```python
from build123d import *

# Parameters (mm, degrees)
F0_R      = 38.1036206278
F1_DEPTH  = 25
F2_COUNT  = 24
F3_DEPTH  = 35
F4_R      = 5
F5_SIZE   = 5
F7_DEPTH  = 50
F8_T      = -2.5
F10_DEPTH = 25
F11_R     = 7.6453811345
F12_DEPTH = 50


with BuildPart() as f1:
    # F0 (on Front) → F1 (new body)
    with BuildSketch(Plane.XZ):
        with BuildLine():
            ThreePointArc((-7.8842675869, 53.139290225), (-35.0884247435, -40.6785974441), (53.721, 0))
            ThreePointArc((53.721, 0), (38.2966086664, 37.6738052983), (0.8807473744, 53.7137796572))
            ThreePointArc((0.8807473744, 53.7137796572), (-3.5135215054, 53.6059792153), (-7.8842675869, 53.139290225))
        make_face()
        Circle(F0_R, mode=Mode.SUBTRACT)
        with BuildLine():
            ThreePointArc((-7.8842675869, 53.139290225), (-3.5135215054, 53.6059792153), (0.8807473744, 53.7137796572))
            ThreePointArc((0.8807473744, 53.7137796572), (0.6904629861, 56.2382962215), (0, 58.674))
            ThreePointArc((0, 58.674), (-1.2045880723, 61.1890122015), (-2.8564405638, 63.4357213824))
            ThreePointArc((-2.8564405638, 63.4357213824), (-4.0797358778, 62.2447411623), (-5.448019844, 63.2658603022))
            ThreePointArc((-5.448019844, 63.2658603022), (-6.792486114, 60.822762014), (-7.6584938023, 58.1720357962))
            ThreePointArc((-7.6584938023, 58.1720357962), (-8.0251266423, 55.6670462968), (-7.8842675869, 53.139290225))
        make_face()
    extrude(amount=F1_DEPTH)


with BuildPart() as f2_1:
    # F2: instance of F1
    add(f1.part.rotate(Axis((0, 0, 0), (0, 1, 0)), 1 * 360 / F2_COUNT))


with BuildPart() as f2_2:
    # F2: instance of F1
    add(f1.part.rotate(Axis((0, 0, 0), (0, 1, 0)), 2 * 360 / F2_COUNT))


with BuildPart() as f2_3:
    # F2: instance of F1
    add(f1.part.rotate(Axis((0, 0, 0), (0, 1, 0)), 3 * 360 / F2_COUNT))


with BuildPart() as f2_4:
    # F2: instance of F1
    add(f1.part.rotate(Axis((0, 0, 0), (0, 1, 0)), 4 * 360 / F2_COUNT))


with BuildPart() as f2_5:
    # F2: instance of F1
    add(f1.part.rotate(Axis((0, 0, 0), (0, 1, 0)), 5 * 360 / F2_COUNT))


with BuildPart() as f2_6:
    # F2: instance of F1
    add(f1.part.rotate(Axis((0, 0, 0), (0, 1, 0)), 6 * 360 / F2_COUNT))


with BuildPart() as f2_7:
    # F2: instance of F1
    add(f1.part.rotate(Axis((0, 0, 0), (0, 1, 0)), 7 * 360 / F2_COUNT))


with BuildPart() as f2_8:
    # F2: instance of F1
    add(f1.part.rotate(Axis((0, 0, 0), (0, 1, 0)), 8 * 360 / F2_COUNT))


with BuildPart() as f2_9:
    # F2: instance of F1
    add(f1.part.rotate(Axis((0, 0, 0), (0, 1, 0)), 9 * 360 / F2_COUNT))


with BuildPart() as f2_10:
    # F2: instance of F1
    add(f1.part.rotate(Axis((0, 0, 0), (0, 1, 0)), 10 * 360 / F2_COUNT))


with BuildPart() as f2_11:
    # F2: instance of F1
    add(f1.part.rotate(Axis((0, 0, 0), (0, 1, 0)), 11 * 360 / F2_COUNT))


with BuildPart() as f2_12:
    # F2: instance of F1
    add(f1.part.rotate(Axis((0, 0, 0), (0, 1, 0)), 12 * 360 / F2_COUNT))


with BuildPart() as f2_13:
    # F2: instance of F1
    add(f1.part.rotate(Axis((0, 0, 0), (0, 1, 0)), 13 * 360 / F2_COUNT))


with BuildPart() as f2_14:
    # F2: instance of F1
    add(f1.part.rotate(Axis((0, 0, 0), (0, 1, 0)), 14 * 360 / F2_COUNT))


with BuildPart() as f2_15:
    # F2: instance of F1
    add(f1.part.rotate(Axis((0, 0, 0), (0, 1, 0)), 15 * 360 / F2_COUNT))


with BuildPart() as f2_16:
    # F2: instance of F1
    add(f1.part.rotate(Axis((0, 0, 0), (0, 1, 0)), 16 * 360 / F2_COUNT))


with BuildPart() as f2_17:
    # F2: instance of F1
    add(f1.part.rotate(Axis((0, 0, 0), (0, 1, 0)), 17 * 360 / F2_COUNT))


with BuildPart() as f2_18:
    # F2: instance of F1
    add(f1.part.rotate(Axis((0, 0, 0), (0, 1, 0)), 18 * 360 / F2_COUNT))


with BuildPart() as f2_19:
    # F2: instance of F1
    add(f1.part.rotate(Axis((0, 0, 0), (0, 1, 0)), 19 * 360 / F2_COUNT))


with BuildPart() as f2_20:
    # F2: instance of F1
    add(f1.part.rotate(Axis((0, 0, 0), (0, 1, 0)), 20 * 360 / F2_COUNT))


with BuildPart() as f2_21:
    # F2: instance of F1
    add(f1.part.rotate(Axis((0, 0, 0), (0, 1, 0)), 21 * 360 / F2_COUNT))


with BuildPart() as f2_22:
    # F2: instance of F1
    add(f1.part.rotate(Axis((0, 0, 0), (0, 1, 0)), 22 * 360 / F2_COUNT))


with BuildPart() as f2_23:
    # F2: instance of F1
    add(f1.part.rotate(Axis((0, 0, 0), (0, 1, 0)), 23 * 360 / F2_COUNT))


with BuildPart() as f1_1:
    add(f1.part)

    add(f2_1.part)  # F3 merges F2_1

    add(f2_2.part)  # F3 merges F2_2

    add(f2_3.part)  # F3 merges F2_3

    add(f2_4.part)  # F3 merges F2_4

    add(f2_5.part)  # F3 merges F2_5

    add(f2_6.part)  # F3 merges F2_6

    add(f2_7.part)  # F3 merges F2_7

    add(f2_8.part)  # F3 merges F2_8

    add(f2_9.part)  # F3 merges F2_9

    add(f2_10.part)  # F3 merges F2_10

    add(f2_11.part)  # F3 merges F2_11

    add(f2_12.part)  # F3 merges F2_12

    add(f2_13.part)  # F3 merges F2_13

    add(f2_14.part)  # F3 merges F2_14

    add(f2_15.part)  # F3 merges F2_15

    add(f2_16.part)  # F3 merges F2_16

    add(f2_17.part)  # F3 merges F2_17

    add(f2_18.part)  # F3 merges F2_18

    add(f2_19.part)  # F3 merges F2_19

    add(f2_20.part)  # F3 merges F2_20

    add(f2_21.part)  # F3 merges F2_21

    add(f2_22.part)  # F3 merges F2_22

    add(f2_23.part)  # F3 merges F2_23
    # F0 (on Front) → F3 (join)
    with BuildSketch(Plane.XZ):
        Circle(F0_R)
        Polygon((22.3287471763, 4.725022344), (19.1299038845, -12.447713203), (4.725022344, -22.3287471763), (-12.447713203, -19.1299038845), (-22.3287471763, -4.725022344), (-19.1299038845, 12.447713203), (-4.725022344, 22.3287471763), (12.447713203, 19.1299038845), align=None, mode=Mode.SUBTRACT)
    extrude(amount=F3_DEPTH)

    # F4
    f4_edges = [f1_1.edges().sort_by_distance(p)[0] for p in [
        (-38.103621, -35, 0),
        (3.861345, -35, 20.729326),
        (17.38823, -35, 11.927463),
        (20.729326, -35, -3.861345),
        (11.927463, -35, -17.38823),
        (-3.861345, -35, -20.729326),
        (-17.38823, -35, -11.927463),
        (-20.729326, -35, 3.861345),
        (-11.927463, -35, 17.38823),
    ]]
    fillet(f4_edges, radius=F4_R)

    # F5
    f5_edges = [f1_1.edges().sort_by_distance(p)[0] for p in [
        (-33.103621, -35, 0),
        (4.776968, -35, 25.644774),
        (-14.755767, -35, 21.51142),
        (21.51142, -35, 14.755767),
        (-25.644774, -35, 4.776968),
        (25.644774, -35, -4.776968),
        (-21.51142, -35, -14.755767),
        (14.755767, -35, -21.51142),
        (-4.776968, -35, -25.644774),
        (36.639155, -33.535534, 0),
        (-38.103621, -30, 0),
        (-23.954189, -33.604656, -5.068985),
        (-20.729326, -30, 3.861345),
        (-20.522483, -33.604656, 13.353856),
        (-11.927463, -30, 17.38823),
        (-5.068985, -33.604656, 23.954189),
        (3.861345, -30, 20.729326),
        (13.353856, -33.604656, 20.522483),
        (17.38823, -30, 11.927463),
        (23.954189, -33.604656, 5.068985),
        (20.729326, -30, -3.861345),
        (20.522483, -33.604656, -13.353856),
        (11.927463, -30, -17.38823),
        (5.068985, -33.604656, -23.954189),
        (-3.861345, -30, -20.729326),
        (-13.353856, -33.604656, -20.522483),
        (-17.38823, -30, -11.927463),
    ]]
    chamfer(f5_edges, length=F5_SIZE)

    # F6 (on Front) → F7 (join)
    with BuildSketch(Plane.XZ):
        with BuildLine():
            ThreePointArc((127.3675560951, -42.6523669827), (27.9093520111, 221.3839321935), (-74.4929984212, -41.5245314744))
            Line((-74.4929984212, -41.5245314744), (-74.4929984212, -70.1153203845))
            Line((-74.4929984212, -70.1153203845), (127.3675560951, -70.1153203845))
            Line((127.3675560951, -70.1153203845), (127.3675560951, -42.6523669827))
        make_face()
    extrude(amount=F7_DEPTH)

    # F8
    f8_openings = [f1_1.faces().sort_by_distance(p)[0] for p in [
        (27.015959, -50, 69.902767),
    ]]
    offset(amount=F8_T, openings=f8_openings, kind=Kind.INTERSECTION)

    # F9 (on face) → F10 (cut)
    with BuildSketch(Plane.XZ.offset(2.5)):
        Polygon((31.7429648501, 47.7299130723), (46.1478463905, 57.6109470455), (49.3466896824, 74.7836825926), (39.4656557091, 89.1885641331), (22.292920162, 92.3874074249), (7.8880386215, 82.5063734516), (4.6891953297, 65.3336379045), (14.570229303, 50.9287563641), align=None)
    extrude(amount=-F10_DEPTH, mode=Mode.SUBTRACT)

    # F11 (on face) → F12 (join)
    with BuildSketch(Plane.XZ.offset(2.5)):
        with Locations((-42.4036420882, 164.3054187298)):
            Circle(F11_R)
    extrude(amount=F12_DEPTH)


solid = f1_1.part
```
Part model, mm, in its own coordinate system. A direction names the side the tool comes from. Round coordinates to 2 decimals unless told otherwise and drop trailing zeros. Loops run counter-clockwise (first coordinate to the right, second up) from the corner with the lowest first, then second, coordinate; pieces in that order, holes last.
1. Slice it at A-A (y = -44.5). Give the cut face in (x, z).
Solutions:
outline: (-74.49, -70.12) - (127.37, -70.12) - (127.37, -42.65) arc R151.07 ccw (long way) to (-74.49, -41.52) - close; circle Ø15.29 at (-42.4, 164.31); hole (-71.99, -67.62) - (124.87, -67.62) - (124.87, -41.52) arc R148.57 ccw (long way) to (-71.99, -40.41) - close
2. Slice it at C-C (x = 145). Give the cut face in (y, z).
Solutions:
outline: (-50, -24.1) - (0, -24.1) - (0, 164.73) - (-50, 164.73) - (-50, 160.67) - (-2.5, 160.67) - (-2.5, -20.04) - (-50, -20.04) - close
3. Slice it at B-B (z = 20.5). Give the cut face in (x, y), and give its area (3 significant figures).
Solutions:
outline: (-115.56, -50) - (-112.9, -50) - (-112.9, -2.5) - (167.04, -2.5) - (167.04, -50) - (169.69, -50) - (169.69, 0) - (-115.56, 0) - close
area: 965 mm2
4. Two-plate mould, pull along X, no slides. Class faces 5 (the face through (-74.493, -25, -56)), 6 (the face through (25, -26, -67.615)), 7 (the face through (25, -25, -70.115)), 8 (the face through (-43.399, -27.15, 171.886)): pulls with the +X half, pulls with the -X half, needs draft (parallel to the pull), parting line crosses it, or undercut.
Solutions:
face 5: pulls with the -X half
face 6: undercut
face 7: needs draft
face 8: undercut
5. Flat gauge pins, fed straight in: pin 1 (8 mm diameter, centred on y = -19.5, z = -54.5, fed in from -X); pin 2 (1.5 mm diameter, centred on y = -41.5, z = 51.5, fed in from +X); pin 3 (1.5 mm diameter, centred on y = -23, z = 109, fed in from -X). Where does each tip first touch, or does it go through?
Solutions:
pin 1: stops at x = -74.49
pin 2: stops at x = 177.05
pin 3: stops at x = -119.17
6. Drill centre lines: line 1 along Z through (x, y) = (23.5, -41); line 2 along X through (y, z) = (-20.5, -43.5); line 3 along Z through (x, y) = (-38, -39.5). Where is each one in solid material? Low to high.
Solutions:
line 1: z = -70.12 to -67.62, 218.84 to 221.34
line 2: x = -74.49 to -71.99, 124.87 to 127.37
line 3: z = -70.12 to -67.62, 158.06 to 170.56, 203.88 to 206.66
7. 3-axis set-ups, long thin cutter, end or side, ignore diameter. For faces 1 (the face through (127.368, -25, -57)), 2 (the face through (25, 0, 45)), 3 (the face through (-71.993, -26, -54)), 4 (the face through (15.191, -1.268, 87.516)): which of +Z, -Z, +X, -X, +Y, -Y reach the whole face in a straight line?
Solutions:
face 1: -Z, +X, +Y, -Y
face 2: +Z, -Z, +X, -X, +Y
face 3: -Y
face 4: +Y, -Y
